Work out the finished part from the listing and answer in its coordinate system (mm). A direction names the side the tool comes from. Coordinates: 2 decimals unless noted, no trailing zeros. Loops run counter-clockwise (first coordinate to the right, second up) from the corner with the lowest first, then second, coordinate; pieces in that order, holes last. Notation, with made-up numbers: (-27.5, -19) -> (-16.5, -19) arc R29 ccw to (-16.5, 15) -> close; hole circle Ø10 at (81.5, -5.5). An arc over 180 degrees is marked (long way). Use a Markdown table: item, result.
from build123d import *

# Parameters (mm, degrees)
F0_W     = 60
F0_H     = 35
F1_DEPTH = 8
F0_W_2   = 50
F0_H_2   = 1.4
F2_DEPTH = 3
F4_DEPTH = 4
F5_DEPTH = 25


with BuildPart() as f1:
    # F0 (on Top) → F1 (new body)
    with BuildSketch(Plane.XY):
        Rectangle(F0_W, F0_H)
        Polygon((-25, -10.9), (-25, -9.5), (25, -9.5), (25, -10.9), (25, -12.5), (25, -14.1), (25, -15.5), (-25, -15.5), (-25, -14.1), (-25, -12.5), align=None, mode=Mode.SUBTRACT)
        Polygon((-25, 10.9), (-25, 12.5), (-25, 14.1), (-25, 15.5), (25, 15.5), (25, 14.1), (25, 12.5), (25, 10.9), (25, 9.5), (-25, 9.5), align=None, mode=Mode.SUBTRACT)
    extrude(amount=F1_DEPTH)

    # F0 (on Top) → F2 (join)
    with BuildSketch(Plane.XY):
        with Locations((0, 14.8)):
            Rectangle(F0_W_2, F0_H_2)
        with Locations((0, 10.2)):
            Rectangle(F0_W_2, F0_H_2)
        with Locations((0, -10.2)):
            Rectangle(F0_W_2, F0_H_2)
        with Locations((0, -14.8)):
            Rectangle(F0_W_2, F0_H_2)
    extrude(amount=F2_DEPTH)

    # F3 (on face) → F4 (cut)
    with BuildSketch(Plane(origin=(0, 0, 0), x_dir=(1, 0, 0), z_dir=(0, 0, -1))):
        with BuildLine():
            ThreePointArc((-14, 6), (-19.1213203436, 8.1213203436), (-17, 3))
            Line((-17, 3), (-17, 4.55))
            ThreePointArc((-17, 4.55), (-18.0253048327, 7.0253048327), (-15.55, 6))
            Line((-15.55, 6), (-14, 6))
        make_face()
        with BuildLine():
            Line((-17, 4.55), (-17, 3))
            ThreePointArc((-17, 3), (-14.8786796564, 3.8786796564), (-14, 6))
            Line((-14, 6), (-15.55, 6))
            ThreePointArc((-15.55, 6), (-15.9746951673, 4.9746951673), (-17, 4.55))
        make_face()
        with BuildLine():
            ThreePointArc((-17, -3), (-19.1213203436, -8.1213203436), (-14, -6))
            Line((-14, -6), (-15.55, -6))
            ThreePointArc((-15.55, -6), (-18.0253048327, -7.0253048327), (-17, -4.55))
            Line((-17, -4.55), (-17, -3))
        make_face()
        with BuildLine():
            Line((-15.55, -6), (-14, -6))
            ThreePointArc((-14, -6), (-14.8786796564, -3.8786796564), (-17, -3))
            Line((-17, -3), (-17, -4.55))
            ThreePointArc((-17, -4.55), (-15.9746951673, -4.9746951673), (-15.55, -6))
        make_face()
        with BuildLine():
            ThreePointArc((14, 6), (14.8786796564, 3.8786796564), (17, 3))
            Line((17, 3), (17, 4.55))
            ThreePointArc((17, 4.55), (15.9746951673, 4.9746951673), (15.55, 6))
            Line((15.55, 6), (14, 6))
        make_face()
        with BuildLine():
            Line((17, 4.55), (17, 3))
            ThreePointArc((17, 3), (19.1213203436, 3.8786796564), (20, 6))
            ThreePointArc((20, 6), (17, 9), (14, 6))
            Line((14, 6), (15.55, 6))
            ThreePointArc((15.55, 6), (17, 7.45), (18.45, 6))
            ThreePointArc((18.45, 6), (18.0253048327, 4.9746951673), (17, 4.55))
        make_face()
        with BuildLine():
            ThreePointArc((17, -3), (14.8786796564, -3.8786796564), (14, -6))
            Line((14, -6), (15.55, -6))
            ThreePointArc((15.55, -6), (15.9746951673, -4.9746951673), (17, -4.55))
            Line((17, -4.55), (17, -3))
        make_face()
        with BuildLine():
            Line((15.55, -6), (14, -6))
            ThreePointArc((14, -6), (17, -9), (20, -6))
            ThreePointArc((20, -6), (19.1213203436, -3.8786796564), (17, -3))
            Line((17, -3), (17, -4.55))
            ThreePointArc((17, -4.55), (18.0253048327, -4.9746951673), (18.45, -6))
            ThreePointArc((18.45, -6), (17, -7.45), (15.55, -6))
        make_face()
    extrude(amount=-F4_DEPTH, mode=Mode.SUBTRACT)

    # F5 (cut): faces of the model
    f5_faces = [f1.faces().sort_by_distance(p)[0] for p in [
        (-17, 6, 0),
        (17, 6, 0),
        (17, -6, 0),
        (-17, -6, 0),
    ]]
    extrude(f5_faces, amount=-F5_DEPTH, mode=Mode.SUBTRACT)


solid = f1.part
Q1. Consider line 1 (Y direction, x = 7.5, z = 7.25); line 2 (X direction, y = 6, z = 2.35); line 3 (Y direction, x = 4.5, z = 1.25). Determine where each line is inside the solid, lowest interval first. Write a range as [from, to].
Solved:
| item | result |
|---|---|
| line 1 | [-17.5, -15.5], [-9.5, 9.5], [15.5, 17.5] |
| line 2 | [-30, -20], [-14, 14], [20, 30] |
| line 3 | [-17.5, -14.1], [-10.9, 10.9], [14.1, 17.5] |
Q2. Section D-D on z = 2 is taken. Determine the outline of the cut face in (x, y), and give its area (3 significant figures).
Solved:
| item | result |
|---|---|
| outline | (-30, -17.5) -> (30, -17.5) -> (30, 17.5) -> (-30, 17.5) -> close; hole (-25, -14.1) -> (25, -14.1) -> (25, -10.9) -> (-25, -10.9) -> close; hole (-25, 10.9) -> (25, 10.9) -> (25, 14.1) -> (-25, 14.1) -> close; hole circle Ø6 at (-17, -6); hole circle Ø6 at (-17, 6); hole circle Ø6 at (17, -6); hole circle Ø6 at (17, 6) |
| area | 1,670 mm² |
Q3. For faces 5 (the flat face through (0, 15, 3)), 6 (the flat face through (0, -17.5, 4)), 7 (the flat face through (0, 14.1, 1)), determine the directions among +Z, -Z, +X, -X, +Y, -Y from which every point of the face is accessible in a straight line to the end or side of a thin tool.
Solved:
| item | result |
|---|---|
| face 5 | +Z |
| face 6 | +Z, -Z, +X, -X, -Y |
| face 7 | +Z, -Z |
Q4. Given pin 1 Ø1.5 at (x, y) = (-9.5, 10.5) entering from +Z; pin 2 Ø1.8 at (x, y) = (16, -7) entering from -Z, each flat-ended and moving along its own axis, determine where each tip first touches the part or whether it passes through.
Solved:
| item | result |
|---|---|
| pin 1 | z = 3 |
| pin 2 | z = 4 |
Q5. Section B-B on x = 4.5 is taken. Determine the outline of the cut face in (y, z).
Solved:
| item | result |
|---|---|
| outline | (-17.5, 0) -> (-14.1, 0) -> (-14.1, 3) -> (-15.5, 3) -> (-15.5, 8) -> (-17.5, 8) -> close; (-10.9, 0) -> (10.9, 0) -> (10.9, 3) -> (9.5, 3) -> (9.5, 8) -> (-9.5, 8) -> (-9.5, 3) -> (-10.9, 3) -> close; (14.1, 0) -> (17.5, 0) -> (17.5, 8) -> (15.5, 8) -> (15.5, 3) -> (14.1, 3) -> close |
Q6. Section C-C on z = 7 is taken. Determine the outline of the cut face in (x, y).
Solved:
| item | result |
|---|---|
| outline | (-30, -17.5) -> (30, -17.5) -> (30, 17.5) -> (-30, 17.5) -> close; hole (-25, -15.5) -> (25, -15.5) -> (25, -9.5) -> (-25, -9.5) -> close; hole (-25, 9.5) -> (25, 9.5) -> (25, 15.5) -> (-25, 15.5) -> close; hole circle Ø2.9 at (-17, -6); hole circle Ø2.9 at (-17, 6); hole circle Ø2.9 at (17, -6); hole circle Ø2.9 at (17, 6) |
Q7. Section A-A on y = 12 is taken. Determine the outline of the cut face in (x, z), and give its area (3 significant figures).
Solved:
| item | result |
|---|---|
| outline | (-30, 0) -> (-25, 0) -> (-25, 8) -> (-30, 8) -> close; (25, 0) -> (30, 0) -> (30, 8) -> (25, 8) -> close |
| area | 80.0 mm² |
Q8. Determine the mould class of faces 1 (the flat face through (0, -15.5, 5)), 2 (the flat face through (30, 0, 4)), 3 (the flat face through (-25, -13, 5)), 4 (the flat face through (0, 17.5, 4)) for opening direction X: pulls with the +X half, pulls with the -X half, needs draft (parallel to the pull), parting line crosses it, or undercut.
Solved:
| item | result |
|---|---|
| face 1 | undercut |
| face 2 | pulls with the +X half |
| face 3 | undercut |
| face 4 | needs draft |
